from build123d import *

# Parameters (mm, degrees)
F0_W     = 12.7
F0_H     = 50.8
F1_DEPTH = 2.54
F3_DEPTH = 12.7
F4_R     = 5.08


with BuildPart() as f1:
    # F0 (on Top) → F1 (new body)
    with BuildSketch(Plane.XY):
        with Locations((6.35, -25.4)):
            Rectangle(F0_W, F0_H)
    extrude(amount=F1_DEPTH)

    # F2 (on face) → F3 (join)
    with BuildSketch(Plane(origin=(0, 0, 0), x_dir=(1, 0, 0), z_dir=(0, 0, -1))):
        Polygon((0, 0), (12.7, 0), (12.7, 2.54), (2.54, 2.54), (2.54, 50.8), (0, 50.8), align=None)
    extrude(amount=F3_DEPTH)

    # F4
    f4_edges = [f1.edges().sort_by_distance(p)[0] for p in [
        (0, 0, -5.08),
        (0, -25.4, 2.54),
        (6.35, 0, 2.54),
    ]]
    fillet(f4_edges, radius=F4_R)


solid = f1.part
Part model, mm, in its own coordinate system. A direction names the side the tool comes from. Give positions to 0.01 mm unless a question says otherwise; leave off trailing zeros. Order: outer loops, then holes, each group sorted by start corner. A loop starts at its lowest first (then second) coordinate and runs counter-clockwise, first axis right, second up. Notation, with made-up numbers: (14.25, 4) - (26.25, 4) arc R17 cw to (26.25, 25) - close; hole circle Ø5 at (32.5, 81.25). An arc over 180 degrees is marked (long way). Use a Markdown table: item, result.
1) Saw through at B-B on z = -8.25. List the corners of the cut face in (x, y), plus the area to 3 significant figures.
Checked values:
| item | result |
|---|---|
| outline | (0, -50.8) - (2.54, -50.8) - (2.54, -2.54) - (12.7, -2.54) - (12.7, 0) - (5.08, 0) arc R5.08 ccw to (0, -5.08) - close |
| area | 149 mm² |
2) Saw through at A-A on y = -36.5. List the corners of the cut face in (x, z), plus the area to 3 significant figures.
Checked values:
| item | result |
|---|---|
| outline | (0, -12.7) - (2.54, -12.7) - (2.54, 0) - (12.7, 0) - (12.7, 2.54) - (5.08, 2.54) arc R5.08 ccw to (0, -2.54) - close |
| area | 59.0 mm² |
3) 3-axis set-ups, long thin cutter, end or side, ignore diameter. For faces 4 (the flat face through (2.54, -26, -6)), 5 (the flat face through (12.7, -23, 1)): which of +Z, -Z, +X, -X, +Y, -Y reach the whole face in a straight line?
Checked values:
| item | result |
|---|---|
| face 4 | -Z, +X, -Y |
| face 5 | +Z, -Z, +X, +Y, -Y |
4) Probe L1, parallel to X at y = -5, z = -7; L2, parallel to Y at x = 5.75, z = -3. List the from-to ranges inside material, lowest first. Write a range as from..to.
Checked values:
| item | result |
|---|---|
| L1 | 0..2.54 |
| L2 | -2.54..0 |
5) Two-plate mould, pull along Z, no slides. Class faces 1 (the flat face through (2, -24, -12.7)), 2 (the cylindrical face through (1.528, -1.449, -7.549)), 3 (the cylindrical face through (1.528, -27.62, 1.091)): +Z half, -Z half, draft (parallel to the pull), parting line (faces both ways), or undercut.
Checked values:
| item | result |
|---|---|
| face 1 | -Z half |
| face 2 | draft |
| face 3 | +Z half |
6) Flat gauge pins, fed straight in: P1, Ø6.5, axis at y = -15.5, z = -6, coming from the +X side; P2, Ø2, axis at y = -17, z = 0.5, coming from the -X side; P3, Ø1.5, axis at x = 8.5, z = 1, coming from the +Y side. Where does each tip first touch, or does it go through?
Checked values:
| item | result |
|---|---|
| P1 | x = 2.54 |
| P2 | x = 0.43 |
| P3 | y = -0.83 |
7) Saw through at C-C on x = 1.25. List the corners of the cut face in (y, z), plus the area to 3 significant figures.
Checked values:
| item | result |
|---|---|
| outline | (-50.8, -12.7) - (-1.74, -12.7) - (-1.74, -2.54) arc R3.34 ccw to (-5.08, 0.8) - (-50.8, 0.8) - close |
| area | 660 mm² |
